Autodesk Inventor part; units mm, degrees
ref_plane "YZ Plane" through (0, 0, 0) normal (1, 0, 0) x (0, 1, 0)
ref_plane "XZ Plane" through (0, 0, 0) normal (0, 1, 0) x (-1, 0, 0)
ref_plane "XY Plane" through (0, 0, 0) normal (0, 0, 1) x (1, 0, 0)
sketch "Sketch1" plane through (0, 0, 0) normal (0, 1, 0) x (-1, 0, 0)
  line L0 (-60, -60) -> (60, -60)
  line L1 (60, -60) -> (60, 60)
  line L2 (60, 60) -> (-60, 60)
  line L3 (-60, 60) -> (-60, -60)
  line L4 (-60, -60) -> (60, 60) construction
  line L5 (60, -60) -> (-60, 60) construction
  line L6 (40, 60) -> (40, 30)
  line L7 (40, 30) -> (50, 30)
  line L8 (50, 30) -> (50, -50)
  line L9 (50, -50) -> (-50, -50)
  line L10 (-50, -50) -> (-50, 30)
  line L11 (-50, 30) -> (-40, 30)
  line L12 (-40, 30) -> (-40, 60)
  point P0 (0, 0)
  dimension "d0" = 120
  dimension "d1" = 120
  dimension "d2" = 20
  dimension "d3" = 20
  dimension "d4" = 10
  dimension "d5" = 10
  dimension "d6" = 10
  dimension "d7" = 30
extrude "Extrusion1" add sketch "Sketch1" along normal blind 40 contours L3 L2 L12 L11 L10 L9 L8 L7 L6 L1 L0
chamfer "Chamfer1" distance 10 angle 45 8 edges at (60, 20, 60) (60, 20, -60) (-50, 20, -50) (-60, 20, -60) (50, 20, -50) (-60, 20, 60) (50, 20, 30) (-50, 20, 30)
sketch "Sketch2" plane through (-60, 0, -50) normal (-1, 0, 0) x (0, 0, 1)
  circle A0 centre (95, 20) radius 10
  line L0 (110, 0) -> (110, 40)
  line L1 (0, 40) -> (100, 40)
  point P0 (50, 0)
  dimension "d13" = 15
  dimension "d14" = 20
  dimension "d15" = 20
extrude "Extrusion2" cut sketch "Sketch2" against normal through all
equation "\"d5\" = d4"
properties part number "frame"
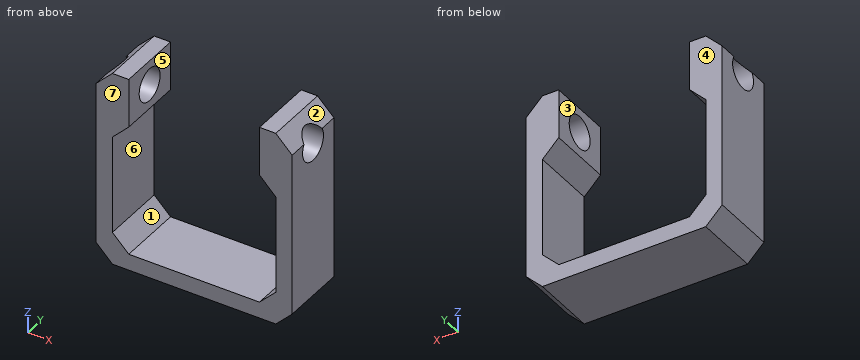
Read the model definition and answer for the solid it produces. Units are mm, in the model's axes. Face numbers are marked on the shaded views. A direction names the side the tool comes from. Coordinates: 2 decimals unless noted, no trailing zeros. Order: outer loops, then holes, each group sorted by start corner. A loop starts at its lowest first (then second) coordinate and runs counter-clockwise, first axis right, second up. Notation, with made-up numbers: M 10,16 L 40,16 A14 ccw 40,32 Z; hole C 59,2.25 d1. An arc over 180 degrees is marked long. Put each result on its own line as item: value. Start each with the question number.
Item 1: Section C-C, the plane z = 45 is taken. Determine the outline of the cut face in (x, y).
Item 2: Section A-A, the plane z = -32 is taken. Determine the outline of the cut face in (x, y).
Item 3: Section B-B, the plane y = 13 is taken. Count the separate pieces of the cut face and the enclosed holes in it, plus the area to 3 significant figures.
Item 4: Given pin 1 Ø1.5 at (x, y) = (31.5, 20) entering from +Z, flat-ended and moving along its own axis, determine where the tip first touches the part or whether it passes through.
Item 5: Consider probe 1 along X at (y, z) = (36.5, 9); probe 2 along Y at (x, z) = (-47, 45); probe 3 along X at (y, z) = (7.5, 31). Determine where each line is inside the solid, lowest interval first. Write a range as [from, to].
Item 6: The mould has two halves that part along X. Classify the marked faces 1, 2, 3 and 4: +X half, -X half, draft (parallel to the pull), parting line (faces both ways), or undercut.
Item 7: For the marked faces 5, 6 and 7, determine the directions among +Z, -Z, +X, -X, +Y, -Y from which every point of the face is accessible in a straight line to the end or side of a thin tool.
Computed:
1. outline: M -60,0 L -40,0 L -40,10 L -60,10 Z; M -60,30 L -40,30 L -40,40 L -60,40 Z; M 40,0 L 60,0 L 60,10 L 40,10 Z; M 40,30 L 60,30 L 60,40 L 40,40 Z
2. outline: M -60,0 L -50,0 L -50,40 L -60,40 Z; M 50,0 L 60,0 L 60,40 L 50,40 Z
3. separate pieces: 3
3. enclosed holes: 0
3. area: 3,430 mm2
4. pin 1: stops at z = -50
5. probe 1: x = [-60, -50], [50, 60]
5. probe 2: y = [0, 10], [30, 40]
5. probe 3: x = [-60, -40], [40, 60]
6. face 1: undercut
6. face 2: +X half
6. face 3: undercut
6. face 4: draft
7. face 5: +Z, +Y, -Y
7. face 6: +Y, -Y
7. face 7: +Z, -Z, +X, -X, -Y
